from build123d import *

# Parameters (mm, degrees)
SKETCH1_R           = 1.5
BOSS_EXTRUDE1_DEPTH = 60
LPATTERN1_COUNT     = 7
LPATTERN1_PITCH     = 1


with BuildPart() as part:
    # Sketch1 → Boss-Extrude1 (new, symmetric)
    with BuildSketch(Plane.XY):
        Circle(SKETCH1_R)
    extrude(amount=BOSS_EXTRUDE1_DEPTH, both=True)

    # Sketch2 → Cut-Revolve1 (revolve, cut)
    with BuildSketch(Plane(origin=(0, 0, 0), x_dir=(0, 0, -1), z_dir=(1, 0, 0)), mode=Mode.PRIVATE) as cut_revolve1_sk:
        Polygon((59.8, -1.5), (59.4, -1.1), (59, -1.5), (59, -1.898251276), (59.8, -1.898251276), align=None)
    cut_revolve1 = revolve(cut_revolve1_sk.sketch.rotate(Axis((0, 0, 60), (0, 0, -1)), 270), axis=Axis((0, 0, 60), (0, 0, -1)), mode=Mode.SUBTRACT)

    # LPattern1: Cut-Revolve1 ×7
    with Locations(*[(0, 0, i * LPATTERN1_PITCH) for i in range(1, LPATTERN1_COUNT)]):
        add(cut_revolve1, mode=Mode.SUBTRACT)

    # Mirror1: Cut-Revolve1 across plane
    add(cut_revolve1.mirror(Plane.XY), mode=Mode.SUBTRACT)

    # Mirror1 copy 1 sketch → Mirror1 copy 1 (revolve, cut)
    with BuildSketch(Plane(origin=(0, 0, -1), x_dir=(0, 0, 1), z_dir=(1, 0, 0))):
        Polygon((59.8, 1.5), (59.4, 1.1), (59, 1.5), (59, 1.898251276), (59.8, 1.898251276), align=None)
    revolve(axis=Axis((0, 0, -61), (0, 0, -1)), mode=Mode.SUBTRACT)

    # Mirror1 copy 2 sketch → Mirror1 copy 2 (revolve, cut)
    with BuildSketch(Plane(origin=(0, 0, -2), x_dir=(0, 0, 1), z_dir=(1, 0, 0))):
        Polygon((59.8, 1.5), (59.4, 1.1), (59, 1.5), (59, 1.898251276), (59.8, 1.898251276), align=None)
    revolve(axis=Axis((0, 0, -62), (0, 0, -1)), mode=Mode.SUBTRACT)

    # Mirror1 copy 3 sketch → Mirror1 copy 3 (revolve, cut)
    with BuildSketch(Plane(origin=(0, 0, -3), x_dir=(0, 0, 1), z_dir=(1, 0, 0))):
        Polygon((59.8, 1.5), (59.4, 1.1), (59, 1.5), (59, 1.898251276), (59.8, 1.898251276), align=None)
    revolve(axis=Axis((0, 0, -63), (0, 0, -1)), mode=Mode.SUBTRACT)

    # Mirror1 copy 4 sketch → Mirror1 copy 4 (revolve, cut)
    with BuildSketch(Plane(origin=(0, 0, -4), x_dir=(0, 0, 1), z_dir=(1, 0, 0))):
        Polygon((59.8, 1.5), (59.4, 1.1), (59, 1.5), (59, 1.898251276), (59.8, 1.898251276), align=None)
    revolve(axis=Axis((0, 0, -64), (0, 0, -1)), mode=Mode.SUBTRACT)

    # Mirror1 copy 5 sketch → Mirror1 copy 5 (revolve, cut)
    with BuildSketch(Plane(origin=(0, 0, -5), x_dir=(0, 0, 1), z_dir=(1, 0, 0))):
        Polygon((59.8, 1.5), (59.4, 1.1), (59, 1.5), (59, 1.898251276), (59.8, 1.898251276), align=None)
    revolve(axis=Axis((0, 0, -65), (0, 0, -1)), mode=Mode.SUBTRACT)

    # Mirror1 copy 6 sketch → Mirror1 copy 6 (revolve, cut)
    with BuildSketch(Plane(origin=(0, 0, -6), x_dir=(0, 0, 1), z_dir=(1, 0, 0))):
        Polygon((59.8, 1.5), (59.4, 1.1), (59, 1.5), (59, 1.898251276), (59.8, 1.898251276), align=None)
    revolve(axis=Axis((0, 0, -66), (0, 0, -1)), mode=Mode.SUBTRACT)


solid = part.part
Geometry: final body of the model. Coordinates: model frame, mm. Round coordinates to 2 decimals unless told otherwise and drop trailing zeros. Order: outer loops, then holes, each group sorted by start corner. A loop starts at its lowest first (then second) coordinate and runs counter-clockwise, first axis right, second up.
Q1. Section A-A, the plane z = 32.5. Output: boundary loops of the cut face in (x, y), and give its area (3 significant figures).
Result sheet:
outline: circle Ø3 at (0, 0)
area: 7.07 mm2
Q2. Pin query (flat end, axial travel): pin 1 (1.5 mm diameter, centred on x = 1, z = -37, fed in from +Y); pin 2 (1 mm diameter, centred on x = 1, z = -22.5, fed in from -Y). Return the tip coordinate at first contact, or that it passes through.
Result sheet:
pin 1: stops at y = 1.48
pin 2: stops at y = -1.41
Q3. Material intervals for probe 1 along X at (y, z) = (0.15, -21); probe 2 along X at (y, z) = (1, -51.5); probe 3 along Y at (x, z) = (-1.1, 7), sorted ascending.
Result sheet:
probe 1: x = -1.49 to 1.49
probe 2: x = -1.12 to 1.12
probe 3: y = -1.02 to 1.02
